Read the model definition and answer for the solid it produces. Units are mm, in the model's axes. A direction names the side the tool comes from. Give positions to 0.01 mm unless a question says otherwise; leave off trailing zeros. Loops run counter-clockwise (first coordinate to the right, second up) from the corner with the lowest first, then second, coordinate; pieces in that order, holes last. Notation, with made-up numbers: (68, 49) - (97, 49) arc R20 ccw to (97, 82) - close; hole circle Ø4 at (40.25, 1). An arc over 180 degrees is marked (long way). Write item = value, one per line.
```python
from build123d import *

# Parameters (mm, degrees)
F0_R      = 22.5
F1_DEPTH  = 5.5
F2_R      = 22.5
F2_R_2    = 2
F3_DEPTH  = 4
F5_DEPTH  = 3
F6_DEPTH  = 7
F8_DEPTH  = 1
F10_DEPTH = 1


with BuildPart() as f1:
    # F0 (on Top) → F1 (new body)
    with BuildSketch(Plane.XY):
        Circle(F0_R)
        with BuildLine():
            Line((-3.75, 14), (3.75, 14))
            Line((3.75, 14), (3.75, 8.3714074526))
            ThreePointArc((3.75, 8.3714074526), (9.3641604002, 4.1755149614), (11.5, -2.5))
            ThreePointArc((11.5, -2.5), (-6.6755149614, -11.8641604002), (-3.75, 8.3714074526))
            Line((-3.75, 8.3714074526), (-3.75, 14))
        make_face(mode=Mode.SUBTRACT)
    extrude(amount=F1_DEPTH)

    # F2 (on face) → F3 (join)
    with BuildSketch(Plane.XY.offset(5.5)):
        Circle(F2_R)
        with Locations((0, -9.7)):
            Circle(F2_R_2, mode=Mode.SUBTRACT)
        with Locations((0, 11)):
            Circle(F2_R_2, mode=Mode.SUBTRACT)
    extrude(amount=F3_DEPTH)

    # F4 (on face) → F5 (join)
    with BuildSketch(Plane.XY.offset(9.5)):
        with BuildLine():
            ThreePointArc((-6, 21.6852484422), (-13.6244265934, -17.9060045795), (22.5, 0))
            ThreePointArc((22.5, 0), (17.9060045795, 13.6244265934), (6, 21.6852484422))
            Line((6, 21.6852484422), (6, 19.6022957839))
            ThreePointArc((6, 19.6022957839), (16.4810497238, 12.1911853402), (20.5, 0))
            ThreePointArc((20.5, 0), (-12.1911853402, -16.4810497238), (-6, 19.6022957839))
            Line((-6, 19.6022957839), (-6, 21.6852484422))
        make_face()
    extrude(amount=F5_DEPTH)

    # F4 (on face) → F6 (join)
    with BuildSketch(Plane.XY.offset(9.5)):
        with BuildLine():
            Line((-0.5, -4.9749371855), (-0.5, 4.9749371855))
            ThreePointArc((-0.5, 4.9749371855), (-5, 0), (-0.5, -4.9749371855))
        make_face()
        with BuildLine():
            ThreePointArc((0.5, -4.9749371855), (3.7080992435, -3.3541019662), (5, 0))
            ThreePointArc((5, 0), (3.7080992435, 3.3541019662), (0.5, 4.9749371855))
            Line((0.5, 4.9749371855), (0.5, -4.9749371855))
        make_face()
    extrude(amount=F6_DEPTH)

    # F7 (on face) → F8 (cut)
    with BuildSketch(Plane.XY.offset(16.5)):
        with BuildLine():
            Line((-0.5, -2.9580398915), (-0.5, 2.9580398915))
            ThreePointArc((-0.5, 2.9580398915), (-3, 0), (-0.5, -2.9580398915))
        make_face()
    extrude(amount=-F8_DEPTH, mode=Mode.SUBTRACT)

    # F9 (on face) → F10 (cut)
    with BuildSketch(Plane.XY.offset(16.5)):
        with BuildLine():
            Line((0.5, 2.9580398915), (0.5, -2.9580398915))
            ThreePointArc((0.5, -2.9580398915), (3, 0), (0.5, 2.9580398915))
        make_face()
    extrude(amount=-F10_DEPTH, mode=Mode.SUBTRACT)


solid = f1.part
```
1) A cutting plane is placed at B-B on z = 11. Determine the outline of the cut face in (x, y).
Output:
outline = (-6, 19.6) - (-6, 21.69) arc R22.5 ccw (long way) to (6, 21.69) - (6, 19.6) arc R20.5 cw (long way) to start; (-0.5, -4.97) - (-0.5, 4.97) arc R5 ccw to start; (0.5, -4.97) arc R5 ccw to (0.5, 4.97) - close
2) A tool of negligible diameter and unlimited length cuts with its end or side. For faces 4 (the face through (-3.75, 11, 3)), 5 (the face through (-0.5, 0, 13)), 6 (the face through (1, 0, 15.5)), from which of +Z, -Z, +X, -X, +Y, -Y can it reach the whole face along a straight path? Write none if from no direction.
Output:
face_4 = -Z
face_5 = +Z, +Y
face_6 = +Z
3) The mould has two halves that part along Y. Classify faces 1 (the face through (15.24, 16.55, 6.16)), 2 (the face through (-1, 0, 15.5)), 3 (the face through (10, 5, 0)): pulls with the +Y half, pulls with the -Y half, needs draft (parallel to the pull), parting line crosses it, or undercut.
Output:
face_1 = parting line crosses it
face_2 = undercut
face_3 = needs draft
4) Find the intervals of material crossed by probe 1 along Y at (x, z) = (0, 4.35); probe 2 along Z at (x, y) = (-13.5, -12.5); probe 3 along Y at (x, z) = (0, 11.4), in increasing order.
Output:
probe_1 = -22.5 to -14, 14 to 22.5
probe_2 = 0 to 9.5
probe_3 = -22.5 to -20.5
5) A cutting plane is placed at C-C on y = -9.7. Determine the outline of the cut face in (x, z), then the cut area to 3 significant figures.
Output:
outline = (-20.3, 0) - (-8.97, 0) - (-8.97, 5.5) - (-2, 5.5) - (-2, 9.5) - (-18.06, 9.5) - (-18.06, 12.5) - (-20.3, 12.5) - close; (2, 5.5) - (8.97, 5.5) - (8.97, 0) - (20.3, 0) - (20.3, 12.5) - (18.06, 12.5) - (18.06, 9.5) - (2, 9.5) - close
area = 285 mm²
6) Each of these flat-tipped pins is pushed along its axis until it touches: P1, Ø1, axis at x = 9, z = 13.5, coming from the +Y side; P2, Ø3, axis at x = -2, z = 3, coming from the -Y side; P3, Ø1.7, axis at y = 21, z = 11.5, coming from the +X side; P4, Ø4.5, axis at y = 11.5, z = 2.5, coming from the +X side. Where does it stop, or does it pass through?
Output:
P1 = through
P2 = -22.49
P3 = 10.01
P4 = 20.51
7) A cutting plane is placed at D-D on x = -12.5. Determine the outline of the cut face in (y, z), then the cut area to 3 significant figures.
Output:
outline = (-18.71, 0) - (18.71, 0) - (18.71, 12.5) - (16.25, 12.5) - (16.25, 9.5) - (-16.25, 9.5) - (-16.25, 12.5) - (-18.71, 12.5) - close
area = 370 mm²
